Source: CAD feature listing. Evaluate the final solid. Frame: model axes, mm. Round coordinates to 2 decimals unless told otherwise and drop trailing zeros. Order: outer loops, then holes, each group sorted by start corner. A loop starts at its lowest first (then second) coordinate and runs counter-clockwise, first axis right, second up. Notation, with made-up numbers: (42, 77) -> (61, 77) arc R27 cw to (61, 112) -> close; hole circle Ø8 at (-21, 10). An arc over 180 degrees is marked (long way). One line per item, written item: value. Start each with the question number.
1) Section C-C (x = 57). Return the cut outline in (y, z).
2) Section B-B (z = -7.5). State how many separate pieces and enclosed holes the cut face has, and give its area (3 significant figures).
3) Pin query (flat end, axial travel): P1, Ø1.7, axis at x = 13.5, y = -29, coming from the +Z side; P2, Ø1.5, axis at x = 57, y = -49.5, coming from the -Z side. Return the tip coordinate at first contact, or that it passes through.
4) Ray query, L1, parallel to X at y = -49, z = -15.5; L2, parallel to X at y = -28.5, z = -2.75; L3, parallel to X at y = -4.5, z = -3.5. Return the intervals inside material, ascending.
5) Section A-A (x = 101). Return the cut outline in (y, z), and give its area (3 significant figures).
```python
from build123d import *

# Parameters (mm, degrees)
F0_R     = 3.175
F1_DEPTH = 22.0345
F2_R     = 2.54
F3_DEPTH = 12.7
F4_R     = 0.3318916447
F4_R_2   = 0.3293568933
F4_R_3   = 0.3316016918
F5_DEPTH = 25.4
F6_R     = 2.778125
F7_DEPTH = 12.7
F9_R     = 4.064


with BuildPart() as f1:
    # F0 (on Top) → F1 (new body)
    with BuildSketch(Plane.XY):
        with BuildLine():
            Line((197.0278, 0), (4.064, 0))
            ThreePointArc((4.064, 0), (1.1903180413, -1.1903180413), (0, -4.064))
            Line((0, -4.064), (0, -51.943))
            ThreePointArc((0, -51.943), (1.1903180413, -54.8166819587), (4.064, -56.007))
            Line((4.064, -56.007), (197.0278, -56.007))
            ThreePointArc((197.0278, -56.007), (199.9014819587, -54.8166819587), (201.0918, -51.943))
            Line((201.0918, -51.943), (201.0918, -4.064))
            ThreePointArc((201.0918, -4.064), (199.9014819587, -1.1903180413), (197.0278, 0))
        make_face()
        with Locations((32.639, -48.60544)):
            Circle(F0_R, mode=Mode.SUBTRACT)
        with Locations((100.5459, -48.60544)):
            Circle(F0_R, mode=Mode.SUBTRACT)
        with Locations((168.5925, -48.60544)):
            Circle(F0_R, mode=Mode.SUBTRACT)
        with Locations((32.639, -7.3914)):
            Circle(F0_R, mode=Mode.SUBTRACT)
        with Locations((100.5713, -7.3914)):
            Circle(F0_R, mode=Mode.SUBTRACT)
        with Locations((168.5925, -7.3914)):
            Circle(F0_R, mode=Mode.SUBTRACT)
    extrude(amount=-F1_DEPTH)

    # F2 (on face) → F3 (cut)
    with BuildSketch(Plane(origin=(0, 0, -22.0345), x_dir=(1, 0, 0), z_dir=(0, 0, -1))):
        with Locations((56.5658, 48.6156)):
            Circle(F2_R)
        with Locations((142.8115, 7.3914)):
            Circle(F2_R)
    extrude(amount=-F3_DEPTH, mode=Mode.SUBTRACT)

    # F4 (on face) → F5 (cut)
    with BuildSketch(Plane.XY):
        with Locations((32.6898, -28.0035)):
            Circle(F4_R)
        with Locations((13.0556, -27.99842)):
            Circle(F4_R_2)
        with Locations((185.039, -28.0035)):
            Circle(F4_R_3)
    extrude(amount=-F5_DEPTH, mode=Mode.SUBTRACT)

    # F6 (on Top) → F7 (cut)
    with BuildSketch(Plane.XY):
        with Locations((185.0457321729, -27.9965074454)):
            Circle(F6_R)
        with Locations((32.6965321729, -27.9965074454)):
            Circle(F6_R)
        with Locations((13.0623321729, -27.9965074454)):
            Circle(F6_R)
    extrude(amount=-F7_DEPTH, mode=Mode.SUBTRACT)

    # F9
    f9_edges = [f1.edges().sort_by_distance(p)[0] for p in [
        (100.5459, -56.007, 0),
        (199.901482, -54.816682, 0),
        (201.0918, -28.0035, 0),
        (199.901482, -1.190318, 0),
        (100.5459, 0, 0),
        (1.190318, -1.190318, 0),
        (0, -28.0035, 0),
        (1.190318, -54.816682, 0),
    ]]
    fillet(f9_edges, radius=F9_R)


solid = f1.part
```
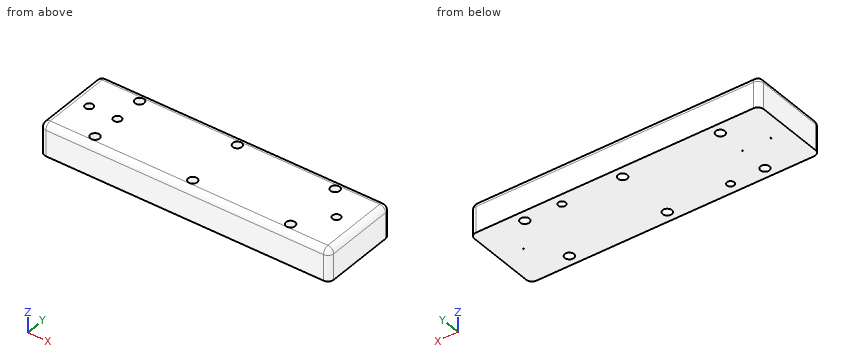
Findings:
1. outline: (-56.01, -22.03) -> (-51.12, -22.03) -> (-51.12, -9.33) -> (-46.11, -9.33) -> (-46.11, -22.03) -> (0, -22.03) -> (0, -4.06) arc R4.06 ccw to (-4.06, 0) -> (-51.94, 0) arc R4.06 ccw to (-56.01, -4.06) -> close
2. separate pieces: 1
2. enclosed holes: 9
2. area: 11,000 mm2
3. P1: z = -12.7
3. P2: z = -9.33
4. L1: 0 to 29.49, 35.79 to 54.06, 59.08 to 97.4, 103.7 to 165.44, 171.74 to 201.09
4. L2: 0.22 to 10.33, 15.79 to 29.96, 35.43 to 182.31, 187.78 to 200.87
4. L3: 0.04 to 31.33, 33.95 to 99.26, 101.88 to 167.28, 169.9 to 201.05
5. outline: (-56.01, -22.03) -> (-51.75, -22.03) -> (-51.75, 0) -> (-51.94, 0) arc R4.06 ccw to (-56.01, -4.06) -> close; (-45.46, -22.03) -> (-10.54, -22.03) -> (-10.54, 0) -> (-45.46, 0) -> close; (-4.25, -22.03) -> (0, -22.03) -> (0, -4.06) arc R4.06 ccw to (-4.06, 0) -> (-4.25, 0) -> close
5. area: 950 mm2
